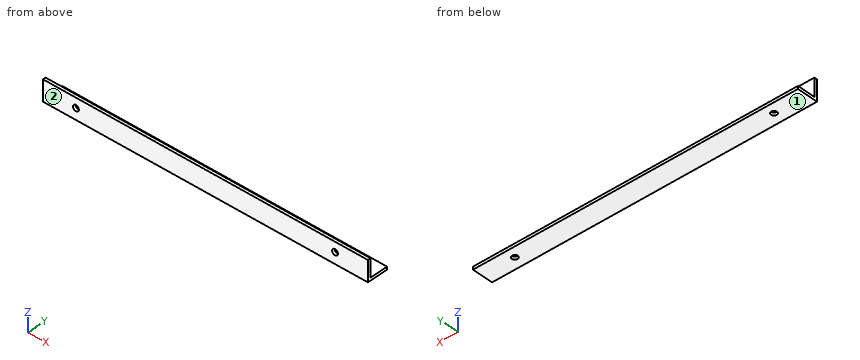
Autodesk Inventor part; units mm, degrees
ref_plane "YZ Plane" through (0, 0, 0) normal (1, 0, 0) x (0, 1, 0)
ref_plane "XZ Plane" through (0, 0, 0) normal (0, 1, 0) x (-1, 0, 0)
ref_plane "XY Plane" through (0, 0, 0) normal (0, 0, 1) x (1, 0, 0)
sketch "Sketch1" plane through (0, 0, 0) normal (0, 0, 1) x (1, 0, 0)
  line L0 (117.25, -7.54) -> (-117.25, -7.54)
  line L1 (-117.25, -7.54) -> (-117.25, 7.54)
  line L2 (-117.25, 7.54) -> (117.25, 7.54)
  line L3 (117.25, 7.54) -> (117.25, -7.54)
  line L4 (117.25, -7.54) -> (-117.25, 7.54) construction
  line L5 (-117.25, -7.54) -> (117.25, 7.54) construction
  point P0 (0, 0)
  dimension "d0" = 234.5
  dimension "d1" = 15.08
extrude "Extrusion1" add sketch "Sketch1" along normal blind 2.05
sketch "Sketch2" plane through (0, 0, 2.05) normal (0, 0, 1) x (1, 0, 0)
  line L0 (-117.25, -7.54) -> (117.25, -7.54)
  line L1 (117.25, -7.54) -> (117.25, 7.54)
  line L2 (-117.25, -7.54) -> (117.25, -7.54)
  line L3 (117.25, -7.54) -> (117.25, -5.49)
  line L4 (117.25, -5.49) -> (-117.25, -5.49)
  line L5 (-117.25, -5.49) -> (-117.25, -7.54)
  point P0 (0, 0)
  dimension "d4" = 2.05
extrude "Extrusion2" add sketch "Sketch2" along normal blind 13.03
sketch "Sketch3" plane through (-117.25, -5.49, 2.05) normal (0, 1, 0) x (1, 0, 0)
  circle A0 centre (23.75, -5.95) radius 2.1
  circle A1 centre (210.75, -5.95) radius 2.1
  line L0 (117.25, 2.05) -> (117.25, -13.2508)
  line L1 (0, 2.05) -> (234.5, 2.05)
  dimension "d7" = 93.5
  dimension "d8" = 93.5
  dimension "d9" = 8
  dimension "d10" = 8
  dimension "d13" = 4.2
  dimension "d14" = 4.2
extrude "Extrusion3" cut sketch "Sketch3" against normal blind 2.05
sketch "Sketch4" plane through (0, 0, 2.05) normal (0, 0, 1) x (1, 0, 0)
  circle A0 centre (-93.5, 0.46) radius 2.1
  circle A1 centre (93.5, 0.46) radius 2.1
  line L0 (-117.25, -7.54) -> (117.25, -7.54)
  point P0 (0, 0)
  dimension "d15" = 4.2
  dimension "d16" = 4.2
  dimension "d17" = 8
  dimension "d18" = 93.5
  dimension "d19" = 93.5
  dimension "d20" = 8
extrude "Extrusion4" cut sketch "Sketch4" against normal blind 2.05
properties part number "L"
Design review of the part built by this model. Coordinates are the model's own, in mm. Face numbers are marked on the shaded views. Round coordinates to 2 decimals unless told otherwise and drop trailing zeros. Write each loop counter-clockwise with the first axis right and the second up, starting at its lowest first coordinate (ties: lowest second). Pieces come first, ordered by that corner, then holes.
Item 1: Consider section D-D on x = 23. Give the boundary of the cut face in (y, z), and give its area (3 significant figures).
Item 2: Consider section B-B on y = 0.46. Give the boundary of the cut face in (x, z).
Item 3: Consider section C-C on x = -93.5. Give the boundary of the cut face in (y, z).
Item 4: Draft analysis for pull direction Z (two halves, no side actions). For the marked faces 1 and 2, state which applies: released by +Z, released by -Z, zero draft, split by the parting line, or undercut.
Item 5: Wall thickness on L1, parallel to X at y = -7, z = 8; L2, parallel to Y at x = 93.5, z = 0.95; L3, parallel to Z at x = -41.5, y = 6.75: over which ranges is each line inside the solid? List them lowest first.
Item 6: For pin 1 Ø6 at (x, y) = (87.5, 3.5) entering from +Z; pin 2 Ø8 at (x, z) = (32, 7) entering from +Y; pin 3 Ø3.5 at (x, y) = (93.5, 0.46) entering from +Z, all flat-tipped, find the tip position at first contact; note any pin that passes through.
Item 7: Consider section A-A on z = 8. Give the boundary of the cut face in (x, y), and give its area (3 significant figures).
Check values:
1. outline: (-7.54, 0) - (7.54, 0) - (7.54, 2.05) - (-5.49, 2.05) - (-5.49, 15.08) - (-7.54, 15.08) - close
1. area: 57.6 mm2
2. outline: (-117.25, 0) - (-95.6, 0) - (-95.6, 2.05) - (-117.25, 2.05) - close; (-91.4, 0) - (91.4, 0) - (91.4, 2.05) - (-91.4, 2.05) - close; (95.6, 0) - (117.25, 0) - (117.25, 2.05) - (95.6, 2.05) - close
3. outline: (-7.54, 0) - (-1.64, 0) - (-1.64, 2.05) - (-5.49, 2.05) - (-5.49, 5.9) - (-7.54, 5.9) - close; (-7.54, 10.1) - (-5.49, 10.1) - (-5.49, 15.08) - (-7.54, 15.08) - close; (2.56, 0) - (7.54, 0) - (7.54, 2.05) - (2.56, 2.05) - close
4. face 1: released by -Z
4. face 2: zero draft
5. L1: x = -117.25 to -95.6, -91.4 to 91.4, 95.6 to 117.25
5. L2: y = -7.54 to -1.64, 2.56 to 7.54
5. L3: z = 0 to 2.05
6. pin 1: stops at z = 2.05
6. pin 2: stops at y = -5.49
6. pin 3: passes through
7. outline: (-117.25, -7.54) - (-95.6, -7.54) - (-95.6, -5.49) - (-117.25, -5.49) - close; (-91.4, -7.54) - (91.4, -7.54) - (91.4, -5.49) - (-91.4, -5.49) - close; (95.6, -7.54) - (117.25, -7.54) - (117.25, -5.49) - (95.6, -5.49) - close
7. area: 464 mm2
